Verification items for the finished model (mm, model axes). Face numbers are marked on the shaded views. Round coordinates to 2 decimals unless told otherwise and drop trailing zeros. Order: outer loops, then holes, each group sorted by start corner. A loop starts at its lowest first (then second) coordinate and runs counter-clockwise, first axis right, second up. Notation, with made-up numbers: M -27,85.5 L 8,85.5 A12 ccw 8,108.5 Z; hole C -28.5,-13.75 d4. An arc over 180 degrees is marked long. Use one line per item in the form item = value. Start each with the question number.
Item 1: Cross-section at D-D on z = 5.75. Enter the section's corners in (x, y), then the cut area to 3 significant figures.
Item 2: Release check for a two-part mould opening along X. For the marked faces 1, 2 and 3 record: +X half, -X half, draft (parallel to the pull), parting line (faces both ways), or undercut.
Item 3: Cross-section at A-A on y = 4.45. Enter the section's corners in (x, z) (3 decimals), then the cut area to 3 significant figures.
Item 4: Thickness scan on probe 1 along X at (y, z) = (4.15, 1.75) (3 decimals); probe 2 along X at (y, z) = (2.4, 8.5); probe 3 along Z at (x, y) = (34.5, 1.95). Record the ranges inside material, lowest first. Write a range as [from, to].
Item 5: Cross-section at C-C on y = 1.55. Enter the section's corners in (x, z) (3 decimals), then the cut area to 3 significant figures.
Item 6: Cross-section at B-B on x = 38. Enter the section's corners in (y, z), then the cut area to 3 significant figures.
Item 7: Go/stop test with flat-tipped pins: pin 1 Ø0.8 at (y, z) = (3.5, 1.5) entering from -X; pin 2 Ø1.1 at (y, z) = (3.5, 20.5) entering from +X; pin 3 Ø3 at (y, z) = (3.5, 19.5) entering from +X; pin 4 Ø2 at (x, y) = (8, 5) entering from -Z. Record where each tip stops, or that it passes through.
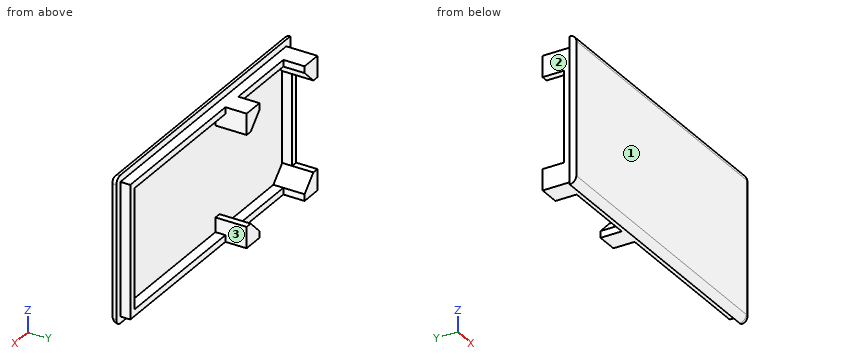
from build123d import *

# Parameters (mm, degrees)
SKETCH1_W                = 43
SKETCH1_H                = 1
BOSS_EXTRUDE1_DEPTH      = 22
FILLET1_R                = 1
SKETCH2_W                = 41
SKETCH2_H                = 20
SKETCH2_W_2              = 39
SKETCH2_H_2              = 18
BOSS_EXTRUDE2_DEPTH      = 1.5
BOSS_EXTRUDE3_DEPTH      = 3.199
BOSS_EXTRUDE3_DEPTH_BACK = 1.5


with BuildPart() as part:
    # Sketch1 → Boss-Extrude1 (new body)
    with BuildSketch(Plane.XY):
        with Locations((21.5, 0.5)):
            Rectangle(SKETCH1_W, SKETCH1_H)
    extrude(amount=BOSS_EXTRUDE1_DEPTH)

    # Fillet1
    # the kernel refuses this fillet: 1 mm, written as the material it takes off along each edge
    with BuildSketch(Plane(origin=(42, 1, 21), x_dir=(1, 0, 0), z_dir=(0, -1, 0))) as fillet1_piece_1_section:
        Polygon((0, 0), (FILLET1_R * 1.02, 0), (FILLET1_R * 1.02, FILLET1_R * 1.02), (0, FILLET1_R * 1.02), align=None)
    fillet1_piece_1 = extrude(amount=FILLET1_R * 1.02, mode=Mode.PRIVATE)
    fillet1_piece_1 = fillet1_piece_1 - Plane(origin=(42, 1, 21), x_dir=(-0.7071067811865475, 0, -0.7071067811865475), z_dir=(0, -1, 0)) * Sphere(FILLET1_R, mode=Mode.PRIVATE)
    add(fillet1_piece_1, mode=Mode.SUBTRACT)
    with BuildSketch(Plane(origin=(42, 1, 1), x_dir=(1, 0, 0), z_dir=(0, -1, 0))) as fillet1_piece_2_section:
        Polygon((0, 0), (FILLET1_R * 1.02, 0), (FILLET1_R * 1.02, -FILLET1_R * 1.02), (0, -FILLET1_R * 1.02), align=None)
    fillet1_piece_2 = extrude(amount=FILLET1_R * 1.02, mode=Mode.PRIVATE)
    fillet1_piece_2 = fillet1_piece_2 - Plane(origin=(42, 1, 1), x_dir=(-0.7071067811865475, 0, 0.7071067811865475), z_dir=(0, -1, 0)) * Sphere(FILLET1_R, mode=Mode.PRIVATE)
    add(fillet1_piece_2, mode=Mode.SUBTRACT)
    with BuildSketch(Plane(origin=(-2.5, 0, 0), x_dir=(0, 0, 1), z_dir=(1, 0, 0))) as fillet1_piece_3:
        with BuildLine():
            CenterArc((FILLET1_R, -FILLET1_R), FILLET1_R, 90, 90)
            Line((0, -FILLET1_R), (0, 0))
            Line((0, 0), (FILLET1_R, 0))
        make_face()
    extrude(amount=44.5, mode=Mode.SUBTRACT)
    with BuildSketch(Plane(origin=(-2.5, 0, 22), x_dir=(0, 0, -1), z_dir=(1, 0, 0))) as fillet1_piece_4:
        with BuildLine():
            CenterArc((FILLET1_R, FILLET1_R), FILLET1_R, 180, 90)
            Line((0, FILLET1_R), (0, 0))
            Line((0, 0), (FILLET1_R, 0))
        make_face()
    extrude(amount=44.5, mode=Mode.SUBTRACT)
    with BuildSketch(Plane(origin=(43, 0, 1), x_dir=(-1, 0, 0), z_dir=(0, 0, 1))) as fillet1_piece_5:
        with BuildLine():
            CenterArc((FILLET1_R, -FILLET1_R), FILLET1_R, 90, 90)
            Line((0, -FILLET1_R), (0, 0))
            Line((0, 0), (FILLET1_R, 0))
        make_face()
    extrude(amount=20, mode=Mode.SUBTRACT)

    # Sketch2 → Boss-Extrude2 (add)
    with BuildSketch(Plane(origin=(0, 1, 0), x_dir=(1, 0, 0), z_dir=(0, 1, 0))):
        with Locations((21.5, -11)):
            Rectangle(SKETCH2_W, SKETCH2_H)
        with Locations((21.5, -11)):
            Rectangle(SKETCH2_W_2, SKETCH2_H_2, mode=Mode.SUBTRACT)
    extrude(amount=BOSS_EXTRUDE2_DEPTH)

    # Sketch3 → Boss-Extrude3 (add, two sides: drawn at the far end of the back side and taken through both)
    with BuildSketch(Plane(origin=(0, 2.5, 0), x_dir=(1, 0, 0), z_dir=(0, 1, 0)).offset(-BOSS_EXTRUDE3_DEPTH_BACK)):
        Polygon((1, -21), (4.175, -21), (4.175, -20), (2, -17.825), (1, -17.825), align=None)
        Polygon((1, -1), (1, -4.175), (2, -4.175), (4.175, -2), (4.175, -1), align=None)
        Polygon((18.494, -21), (18.494, -17.825), (17.494, -17.825), (15.319, -20), (15.319, -21), align=None)
        Polygon((18.494, -1), (18.494, -4.175), (17.494, -4.175), (15.319, -2), (15.319, -1), align=None)
    extrude(amount=BOSS_EXTRUDE3_DEPTH + BOSS_EXTRUDE3_DEPTH_BACK)


solid = part.part
Output values:
q1.outline = M 0,0 L 42,0 A1 ccw 43,1 L 42,1 L 42,2.5 L 41,2.5 L 41,1 L 2,1 L 2,2.5 L 1,2.5 L 1,1 L 0,1 Z
q1.area = 45.8 mm2
q2.face_1 = draft
q2.face_2 = -X half
q2.face_3 = undercut
q3.outline = M 1,1 L 4.175,1 L 4.175,2 L 2,4.175 L 1,4.175 Z; M 1,17.825 L 2,17.825 L 4.175,20 L 4.175,21 L 1,21 Z; M 15.319,1 L 18.494,1 L 18.494,4.175 L 17.494,4.175 L 15.319,2 Z; M 15.319,20 L 17.494,17.825 L 18.494,17.825 L 18.494,21 L 15.319,21 Z
q3.area = 30.9 mm2
q4.probe_1 = [1, 4.175], [15.319, 18.494]
q4.probe_2 = [1, 2], [41, 42]
q4.probe_3 = [1, 2], [20, 21]
q5.outline = M 1,1 L 42,1 L 42,21 L 1,21 Z; hole M 2,4.175 L 4.175,2 L 15.319,2 L 17.494,4.175 L 18.494,4.175 L 18.494,2 L 41,2 L 41,20 L 18.494,20 L 18.494,17.825 L 17.494,17.825 L 15.319,20 L 4.175,20 L 2,17.825 Z
q5.area = 132 mm2
q6.outline = M 0,1 A1 ccw 1,0 L 1,1 L 2.5,1 L 2.5,2 L 1,2 L 1,20 L 2.5,20 L 2.5,21 L 1,21 L 1,22 A1 ccw 0,21 Z
q6.area = 24.6 mm2
q7.pin_1 = 1
q7.pin_2 = 18.49
q7.pin_3 = 42
q7.pin_4 = through
